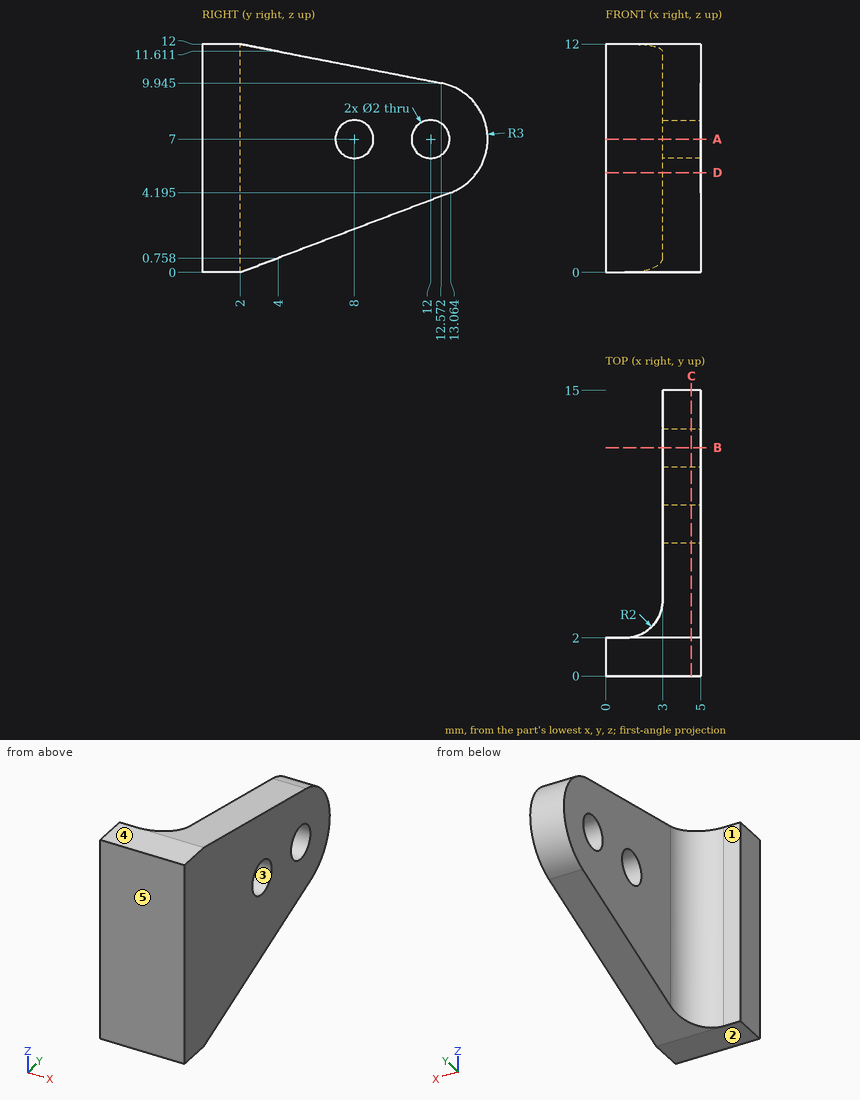
Study the drawing (mm; zero at the part's minimum x, y, z) and answer. A direction names the side the tool comes from. Give positions to 0.01 mm unless a question says otherwise; leave off trailing zeros. Write each loop counter-clockwise with the first axis right and the second up, starting at its lowest first coordinate (ties: lowest second). Pieces come first, ordered by that corner, then holes. Notation, with made-up numbers: (-2, -0.5) -> (22, -0.5) arc R31 cw to (22, 36.5) -> close; hole circle Ø3 at (11, 36). An arc over 180 degrees is marked (long way). Write item = value, one per line.
Q1. Consider line 1 along Y through (x, z) = (3.6, 7); line 2 along Y through (x, z) = (0.7, 4.5); line 3 along X through (y, z) = (8.5, 5.5). Determine where each line is inside the solid, lowest interval first.
Computed values:
line_1 = 0 to 7, 9 to 11, 13 to 15
line_2 = 0 to 2
line_3 = 3 to 5
Q2. Section A-A on z = 7 is taken. Determine the outline of the cut face in (x, y).
Computed values:
outline = (0, 0) -> (5, 0) -> (5, 7) -> (3, 7) -> (3, 4) arc R2 cw to (1, 2) -> (0, 2) -> close; (3, 9) -> (5, 9) -> (5, 11) -> (3, 11) -> close; (3, 13) -> (5, 13) -> (5, 15) -> (3, 15) -> close
Q3. Section B-B on y = 12 is taken. Determine the outline of the cut face in (x, z).
Computed values:
outline = (3, 3.79) -> (5, 3.79) -> (5, 6) -> (3, 6) -> close; (3, 8) -> (5, 8) -> (5, 10.06) -> (3, 10.06) -> close
Q4. Flat-ended cylindrical pins translate along their axes: pin 1 Ø3 at (y, z) = (12, 7) entering from -X; pin 2 Ø1.1 at (x, z) = (0.5, 3.5) entering from +Y. Find the tip coordinate at first contact, or state that the pin passes through.
Computed values:
pin_1 = 3
pin_2 = 2
Q5. Section D-D on z = 5.25 is taken. Determine the outline of the cut face in (x, y).
Computed values:
outline = (0, 0) -> (5, 0) -> (5, 14.44) -> (3, 14.44) -> (3, 4) arc R2 cw to (1, 2) -> (0, 2) -> close
Q6. For a pull along Y with two mould halves and no side action, classify the marked faces 3, 4 and 5 as pulls with the +Y half, pulls with the -Y half, needs draft (parallel to the pull), parting line crosses it, or undercut.
Computed values:
face_3 = undercut
face_4 = needs draft
face_5 = pulls with the -Y half
Q7. A tool of negligible diameter and unlimited length cuts with its end or side. For the marked faces 1 and 2, from which of +Z, -Z, +X, -X, +Y, -Y can it reach the whole face along a straight path? Write none if from no direction.
Computed values:
face_1 = +Z, -Z, -X, +Y
face_2 = -Z, +X, -X, +Y, -Y
Q8. Section C-C on x = 4.5 is taken. Determine the outline of the cut face in (y, z) (1 decimal).
Computed values:
outline = (0, 0) -> (2, 0) -> (13.1, 4.2) arc R3 ccw to (12.6, 9.9) -> (2, 12) -> (0, 12) -> close; hole circle Ø2 at (8, 7); hole circle Ø2 at (12, 7)
